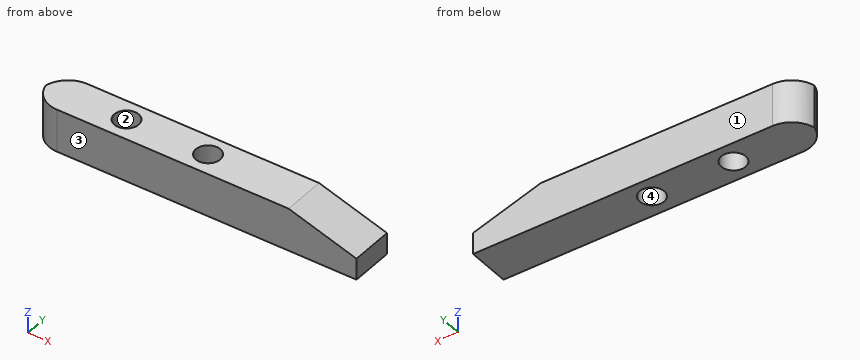
```python
from build123d import *

# Parameters (mm, degrees)
F1_DEPTH    = 16.002
F3_D        = 9.144
F4_T1_DEPTH = 66.802


# Not quite as in the source:
# - a fillet or chamfer that OpenCascade refuses, or shapes differently, is made with other operations: its cross-section is extruded or revolved along the edge and cut away or added


with BuildPart() as f1:
    # F0 (on Front) → F1 (new body)
    with BuildSketch(Plane.XZ):
        Polygon((58.8562823832, 9.8717374111), (-37.9177176168, 9.8717374111), (-37.9177176168, -6.1302625889), (84.2562823832, -6.1302625889), (84.2562823832, 1.8707374111), align=None)
    extrude(amount=F1_DEPTH)

    # F3 (through all)
    with Locations(Plane.XY.offset(9.8717374111)):
        with Locations((-7.6279942878, -7.7707557939), (22.8794198483, -7.7707557939)):
            Hole(F3_D / 2)

    # F4: fillet of radius 10.16 on 2 edges, made by hand

    # F4_s2 → F4_t1 (cut)
    with BuildSketch(Plane.XY.offset(-31.5302625889)):
        with BuildLine():
            ThreePointArc((-27.7577176168, -16.002), (-34.9419225137, -13.0262048969), (-37.9177176168, -5.842))
            Line((-37.9177176168, -5.842), (-37.9177176168, -16.002))
            Line((-37.9177176168, -16.002), (-27.7577176168, -16.002))
        make_face()
        with BuildLine():
            ThreePointArc((-27.7577176168, 0), (-34.9419225137, -2.9757951031), (-37.9177176168, -10.16))
            Line((-37.9177176168, -10.16), (-37.9177176168, 0))
            Line((-37.9177176168, 0), (-27.7577176168, 0))
        make_face()
    extrude(amount=F4_T1_DEPTH, mode=Mode.SUBTRACT)


solid = f1.part
```
Can you work these out from the model? Positions are in its coordinate system, mm. Face numbers are marked on the shaded views. Give positions to 0.01 mm unless a question says otherwise; leave off trailing zeros. Loops run counter-clockwise (first coordinate to the right, second up) from the corner with the lowest first, then second, coordinate; pieces in that order, holes last. Notation, with made-up numbers: M 89.5,-1 L 119.5,-1 A31 cw 119.5,23 Z; hole C 63.5,10.25 d7. An arc over 180 degrees is marked long. One line per question, with ' | ' between items. Start each with the question number.
Q1. If we section it at B-B (z = 7.75): Please give me the cut outline in (x, y), plus the area to 3 significant figures.
Q2. For pin 1 Ø3 at (x, y) = (63, -12.5) entering from +Z; pin 2 Ø5 at (y, z) = (-4, 3) entering from +X, each with a flat end and sliding along its axis, tell me the tip position at first contact or that it passes through.
Q3. If we section it at C-C (y = -11): Please give me the cut outline in (x, z).
Q4. If we mould it in two halves opening along Y, with no side actions, what happens to the marked faces 1, 2, 3 and 4? For each: +Y half, -Y half, draft (parallel to the pull), parting line (faces both ways), or undercut.
Q5. If we section it at D-D (z = -3.25): Please give me the cut outline in (x, y), plus the area to 3 significant figures.
Q6. If we section it at A-A (y = -5.25): Please give me the cut outline in (x, z), plus the area to 3 significant figures.
Q7. If I drill on line 1 (X direction, y = -5.25, z = -4.25); line 2 (X direction, y = -5, z = 0.75); line 3 (Y direction, x = 22.5, z = -0.5), over which ranges is the centre line in solid material (lowest first)? Write a range as from..to.
Computed:
1) outline: M -37.69,-8 A10.16 ccw -27.76,-16 L 65.59,-16 L 65.59,0 L -27.76,0 A10.16 ccw Z; hole C -7.63,-7.77 d9.14; hole C 22.88,-7.77 d9.14 | area: 1,480 mm²
2) pin 1: stops at z = 9.04 | pin 2: stops at x = 84.26
3) outline: M -36.51,-6.13 L -10.86,-6.13 L -10.86,9.87 L -36.51,9.87 Z; M -4.39,-6.13 L 19.64,-6.13 L 19.64,9.87 L -4.39,9.87 Z; M 26.12,-6.13 L 84.26,-6.13 L 84.26,1.87 L 58.86,9.87 L 26.12,9.87 Z
4) face 1: +Y half | face 2: undercut | face 3: -Y half | face 4: undercut
5) outline: M -37.69,-8 A10.16 ccw -27.76,-16 L 84.26,-16 L 84.26,0 L -27.76,0 A10.16 ccw Z; hole C -7.63,-7.77 d9.14; hole C 22.88,-7.77 d9.14 | area: 1,780 mm²
6) outline: M -36.65,-6.13 L -11.44,-6.13 L -11.44,9.87 L -36.65,9.87 Z; M -3.81,-6.13 L 19.07,-6.13 L 19.07,9.87 L -3.81,9.87 Z; M 26.69,-6.13 L 84.26,-6.13 L 84.26,1.87 L 58.86,9.87 L 26.69,9.87 Z | area: 1,590 mm²
7) line 1: x = -36.65..-11.44, -3.81..19.07, 26.69..84.26 | line 2: x = -36.51..-11.26, -3.99..19.24, 26.52..84.26 | line 3: y = -16..-12.33, -3.21..0
